Input: part model. Units: mm. Frame: model coordinates. Face numbers are marked on the shaded views. A direction names the side the tool comes from. Coordinates: 2 decimals unless noted, no trailing zeros. Order: outer loops, then holes, each group sorted by start corner. A loop starts at its lowest first (then second) coordinate and runs counter-clockwise, first axis right, second up. Notation, with made-up numbers: (57.25, 89) - (110.25, 89) arc R22 cw to (110.25, 118) - close; hole circle Ø6 at (81.25, -29.5). An arc over 180 degrees is marked (long way). Use a Markdown table: item, result. Add a question column.
from build123d import *

# Parameters (mm, degrees)
SKETCH8_R             = 6.35
BOSS_EXTRUDE7_DEPTH   = 19.05
SKETCH8_R_2           = 15.875
BOSS_EXTRUDE7_2_DEPTH = 19.05
SKETCH8_R_3           = 5.55625
BOSS_EXTRUDE7_3_DEPTH = 19.05
BOSS_EXTRUDE8_DEPTH   = 12.7
SKETCH9_R             = 3.175
SKETCH9_R_2           = 12.7
SKETCH9_R_3           = 2.38125
CUT_EXTRUDE3_DEPTH    = 67.556631241
SHELL3_START          = 3.175
SHELL3_DEPTH          = 9.525
SKETCH11_R            = 15.875
BOSS_EXTRUDE9_DEPTH   = 19.05
SKETCH12_R            = 3.96875
SKETCH12_R_2          = 11.1125
SKETCH12_R_3          = 3.175
CUT_EXTRUDE4_DEPTH    = 67.556631241
FILLET1_R             = 1.905


# Read off the part's stored shape, not the designer's step: Shell3
with BuildPart() as part:
    # Sketch8 → Boss-Extrude7 (new body)
    with BuildSketch(Plane(origin=(0, 0, 0), x_dir=(1, 0, 0), z_dir=(0, 1, 0))):
        with Locations(Location((-44.45, 0, 0), (0, 0, 90))):
            Circle(SKETCH8_R)
    extrude(amount=BOSS_EXTRUDE7_DEPTH)



with BuildPart() as body_2:
    # Sketch8 → Boss-Extrude7 2 (new body)
    with BuildSketch(Plane(origin=(0, 0, 0), x_dir=(1, 0, 0), z_dir=(0, 1, 0))):
        with Locations(Location((0, 0, 0), (0, 0, 90))):
            Circle(SKETCH8_R_2)
    extrude(amount=BOSS_EXTRUDE7_2_DEPTH)


with BuildPart() as body_3:
    # Sketch8 → Boss-Extrude7 3 (new body)
    with BuildSketch(Plane(origin=(0, 0, 0), x_dir=(1, 0, 0), z_dir=(0, 1, 0))):
        with Locations(Location((19.05, -32.995567884, 0), (0, 0, 90))):
            Circle(SKETCH8_R_3)
    extrude(amount=BOSS_EXTRUDE7_3_DEPTH)


with BuildPart() as part_1:
    add(part.part)

    add(body_2.part)  # Boss-Extrude8 merges body 2

    add(body_3.part)  # Boss-Extrude8 merges body 3
    # Sketch1 → Boss-Extrude8 (add)
    with BuildSketch(Plane(origin=(0, 0, 0), x_dir=(1, 0, 0), z_dir=(0, 1, 0))):
        with BuildLine():
            ThreePointArc((15.874516986, 0.123836405), (15.874879246, 0.061918673), (15.875, 0))
            ThreePointArc((15.875, 0), (-8.083566746, -13.662780598), (-7.642678571, 13.914204586))
            ThreePointArc((-7.642678571, 13.914204586), (-25.197394313, 7.419323178), (-43.883035714, 6.324638448))
            ThreePointArc((-43.883035714, 6.324638448), (-39.763704917, 4.284989894), (-38.1, 0))
            ThreePointArc((-38.1, 0), (-39.80230939, -4.326831634), (-43.996526612, -6.333787326))
            ThreePointArc((-43.996526612, -6.333787326), (-10.719971263, -13.048717363), (14.342154608, -35.946517871))
            ThreePointArc((14.342154608, -35.946517871), (16.221269303, -28.213288437), (23.903541316, -30.290932834))
            ThreePointArc((23.903541316, -30.290932834), (17.975858999, -15.588595272), (15.874516986, 0.123836405))
        make_face()
    extrude(amount=BOSS_EXTRUDE8_DEPTH)

    # Sketch9 → Cut-Extrude3 (cut, through all)
    with BuildSketch(Plane(origin=(0, 19.05, 0), x_dir=(1, 0, 0), z_dir=(0, 1, 0))):
        with Locations(Location((-44.45, 0, 0), (0, 0, 270))):
            Circle(SKETCH9_R)
        with Locations(Location((0, 0, 0), (0, 0, 270))):
            Circle(SKETCH9_R_2)
        with Locations(Location((19.05, -32.995567884, 0), (0, 0, 270))):
            Circle(SKETCH9_R_3)
    extrude(amount=-CUT_EXTRUDE3_DEPTH, mode=Mode.SUBTRACT)

    # Shell3 outline → Shell3 (cut)
    with BuildSketch(Plane(origin=(0, 0, 0), x_dir=(1, 0, 0), z_dir=(0, 1, 0)).offset(SHELL3_START)):
        with BuildLine():
            ThreePointArc((-38.800169089, 2.898604954), (-38.1002552, -0.05692953), (-38.853048837, -2.999439561))
            ThreePointArc((-38.853048837, -2.999439561), (-25.959917491, -4.378054539), (-13.577434664, -8.226110438))
            ThreePointArc((-13.577434664, -8.226110438), (-15.868541202, -0.452796995), (-14.024412997, 7.438512289))
            ThreePointArc((-14.024412997, 7.438512289), (-26.19595995, 3.987969239), (-38.800169089, 2.898604954))
        make_face()
        with BuildLine():
            ThreePointArc((13.339048882, -8.607287606), (7.563042072, -13.957650935), (-0.073256974, -15.874830973))
            ThreePointArc((-0.073256974, -15.874830973), (7.639502671, -22.480309716), (14.259701701, -30.180437999))
            ThreePointArc((14.259701701, -30.180437999), (16.221269303, -28.213288437), (18.889968849, -27.441622971))
            ThreePointArc((18.889968849, -27.441622971), (15.417387842, -18.229913189), (13.339048882, -8.607287606))
        make_face()
    extrude(amount=SHELL3_DEPTH, mode=Mode.SUBTRACT)

    # Sketch11 → Boss-Extrude9 (add)
    with BuildSketch(Plane(origin=(0, 0, 0), x_dir=(1, 0, 0), z_dir=(0, 1, 0))):
        with Locations(Location((0, 0, 0), (0, 0, 118.778745897))):
            Circle(SKETCH11_R)
    extrude(amount=BOSS_EXTRUDE9_DEPTH)

    # Sketch12 → Cut-Extrude4 (cut, through all)
    with BuildSketch(Plane(origin=(0, 19.05, 0), x_dir=(1, 0, 0), z_dir=(0, 1, 0))):
        with Locations(Location((-44.45, 0, 0), (0, 0, 270))):
            Circle(SKETCH12_R)
        with Locations(Location((0, 0, 0), (0, 0, 270))):
            Circle(SKETCH12_R_2)
        with Locations(Location((19.05, -32.995567884, 0), (0, 0, 270))):
            Circle(SKETCH12_R_3)
    extrude(amount=-CUT_EXTRUDE4_DEPTH, mode=Mode.SUBTRACT)

    # Fillet1
    fillet1_edges = [part_1.edges().sort_by_distance(p)[0] for p in [
        (18.889968849, 7.9375, 27.441622971),
        (14.259701701, 7.9375, 30.180437999),
        (-0.073256974, 7.9375, 15.874830973),
        (13.339048882, 7.9375, 8.607287606),
        (-14.024412997, 7.9375, -7.438512289),
        (-13.577434664, 7.9375, 8.226110438),
        (-38.800169089, 7.9375, -2.898604954),
        (-38.853048837, 7.9375, 2.999439561),
    ]]
    fillet(fillet1_edges, radius=FILLET1_R)


solid = part_1.part
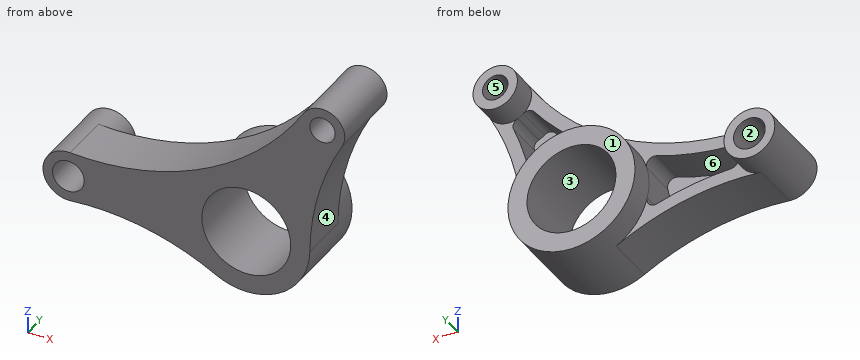
1) Material intervals for L1, parallel to X at y = 9.5, z = 0 (1 decimal); L2, parallel to X at y = 18, z = -2; L3, parallel to X at y = 17.25, z = 8.5, sorted ascending.
2) Reachability of the marked faces 5 and 6 from +Z, -Z, +X, -X, +Y, -Y: full face, straight path, thin tool, end or side. Return the list, or none.
3) Cut plane A-A (z = -9.5). Return the cut outline in (x, y), and give its area (3 significant figures).
4) Cut plane D-D (z = 23). Return the cut outline in (x, y) (1 decimal).
5) Pull-direction query (Z, two-part tool) for the marked faces 1, 2, 3 and 4; classes: pulls with the +Z half, pulls with the -Z half, needs draft (parallel to the pull), parting line crosses it, or undercut.
6) Contact query for flat-ended pins moving along their axis: P1, Ø8, axis at x = -10, y = 3, coming from the -Z side; P2, Ø6, axis at x = -35, y = 8, coming from the -Z side; P3, Ø1, axis at y = 15, z = 2.5, coming from the -X side. Output: stop coordinate, or through.
7) Cut plane B-B (x = 19.05). Return the cut outline in (y, z).
8) Cut plane C-C (x = -25.5). Return the cut outline in (y, z) (3 decimals).
Computed:
| question | item | result |
|---|---|---|
| 1 | L1 | x = -50.8 to -48.4, -40.5 to -38.1, -15.9 to -11.1, 11.1 to 15.9 |
| 1 | L2 | x = -50.48 to -47.88, -41.02 to -38.42, -15.75 to -10.93, 10.93 to 15.75 |
| 1 | L3 | x = -13.41 to -7.16, 7.16 to 13.41 |
| 2 | face 5 | +Y, -Y |
| 2 | face 6 | +Y |
| 3 | outline | (-17.63, 0) - (-5.77, 0) - (-5.77, 19.05) - (-12.72, 19.05) - (-12.72, 12.7) - (-17.63, 12.7) - close; (5.77, 0) - (12.72, 0) - (12.72, 19.05) - (5.77, 19.05) - close |
| 3 | area | 327 mm2 |
| 4 | outline | (3.6, 0) - (20.4, 0) - (20.4, 12.7) - (17, 12.7) - (17, 3.2) - (8.2, 3.2) - (8.2, 12.7) - (3.6, 12.7) - close |
| 5 | face 1 | needs draft |
| 5 | face 2 | undercut |
| 5 | face 3 | undercut |
| 5 | face 4 | pulls with the -Z half |
| 6 | P1 | stops at z = -14.7 |
| 6 | P2 | stops at z = -6.38 |
| 6 | P3 | stops at x = -50.48 |
| 7 | outline | (0, 19.22) - (12.7, 19.22) - (12.7, 27.44) - (19.05, 27.44) - (19.05, 29.82) - (0, 29.82) - close; (0, 36.17) - (19.05, 36.17) - (19.05, 38.55) - (0, 38.55) - close |
| 8 | outline | (0, -7.357) - (12.7, -7.357) - (12.7, -4.119) - (3.175, -4.119) - (3.175, 4.475) - (12.7, 4.475) - (12.7, 7.726) - (0, 7.726) - close |
